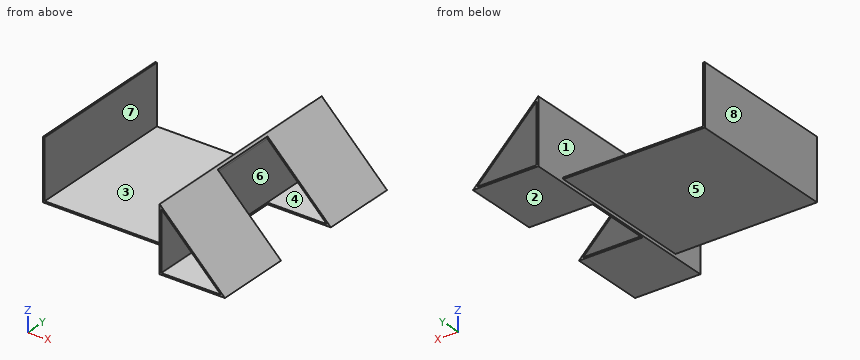
Autodesk Fusion 360 part; units mm, degrees
sketch "Sketch1" plane through (0, 0, 0) normal (0, 1, 0) x (1, 0, 0)
  line L0 (0, 0) -> (-2, 0)
  line L1 (-2, 0) -> (-2, -72)
  line L2 (-2, -72) -> (0, -72)
  line L3 (0, -72) -> (0, 0)
  line L4 (0, 0) -> (166, 0)
  line L5 (166, 0) -> (166, -2)
  line L6 (166, -2) -> (0, -2)
  line L7 (0, -2) -> (0, 0)
  line L8 (166, -72.909) -> (166, 4.011)
  line L9 (166, -72.909) -> (243.52, 4.011)
  line L10 (166, 4.011) -> (243.52, 4.011)
  line L11 (168, -68.107) -> (238.6649, 2.011)
  line L12 (168, 2.011) -> (238.6649, 2.011)
  line L13 (168, -68.107) -> (168, 2.011)
  dimension "d1" = 2
  dimension "d2" = 72
  dimension "d3" = 166
  dimension "d4" = 2
  dimension "d5" = 76.92
  dimension "d6" = 4.011
  dimension "d8" = 77.52
  dimension "d9" = 2
extrude "Extrude1" add sketch "Sketch1" along normal blind 260
sketch "Sketch2" plane through (0, 0, 2) normal (0, 0, 1) x (-1, 0, 0)
  line L0 (0, 0) -> (-166, 0)
  line L1 (-166, 0) -> (-166, -260)
  line L2 (-166, -260) -> (0, -260)
  line L3 (0, -260) -> (0, 0)
  line L4 (2, 0) -> (-166, 0)
  line L5 (-166, 0) -> (-166, -40)
  line L6 (-166, -40) -> (2, -40)
  line L7 (2, -40) -> (2, 0)
  line L8 (0, -130) -> (-166, -130) construction
  line L9 (2, -220) -> (2, -260)
  line L10 (-166, -220) -> (2, -220)
  line L11 (2, -260) -> (-166, -260)
  line L12 (-166, -260) -> (-166, -220)
  point P0 (2, 0)
  dimension "d12" = 168
  dimension "d13" = 40
extrude "Extrude2" cut sketch "Sketch2" against normal blind 45 contours L0 L1 L3 L4 L5 L6 | L3 L4 L6 L7 | L3 L9 L10 L11 | L1 L2 L3 L10 L11 L12
extrude "Extrude3" cut sketch "Sketch2" along normal blind 80 contours L3 L4 L6 L7 | L3 L9 L10 L11
sketch "Sketch3" plane through (0, 0, 2) normal (0, 0, 1) x (-1, 0, 0)
  line L0 (-166, -220) -> (0, -220)
  line L1 (0, -220) -> (0, -40)
  line L2 (0, -40) -> (-166, -40)
  line L3 (-166, -40) -> (-166, -220)
  line L4 (-168.32, -170) -> (-243.52, -170)
  line L5 (-243.52, -170) -> (-243.52, -90)
  line L6 (-243.52, -90) -> (-168.32, -90)
  line L7 (-168.32, -90) -> (-168.32, -170)
  line L8 (-243.52, 0) -> (-243.52, -260)
  dimension "d18" = 75.2
  dimension "d19" = 80
extrude "Extrude4" cut sketch "Sketch3" along normal mid plane 260 contours L4 L5 L6 L7 L8
equation "d2 = ( 7.2 * 10 ) * 1 mm"
equation "d3 = ( 16.6 * 10 ) * 1 mm"
Model file for the job. Use its own axes, mm. Face numbers are marked on the shaded views. A direction names the side the tool comes from. Give positions to 0.01 mm unless a question says otherwise; leave off trailing zeros. Loops run counter-clockwise (first coordinate to the right, second up) from the corner with the lowest first, then second, coordinate; pieces in that order, holes last. Notation, with made-up numbers: (70.25, 88) -> (86.25, 88) arc R20 cw to (86.25, 105) -> close; hole circle Ø8 at (-37, 62). An arc over 180 degrees is marked (long way). Use a Markdown table: item, result. Add a question column.
(1) Tool access for the marked faces 5, 6, 7 and 8: list every direction of +Z, -Z, +X, -X, +Y, -Y with a clear straight run to the whole face (end or side of a thin tool).
(2) Drop flat-ended pins along their axis: pin 1 Ø1 at (y, z) = (100, 9) entering from +X; pin 2 Ø1 at (x, y) = (-1, 114.5) entering from +Z; pin 3 Ø1 at (y, z) = (119, -3) entering from +X; pin 4 Ø22.5 at (x, z) = (213.5, 30) entering from +Y. Give the stop position or say it passes through.
(3) Slice it at A-A on y = 43. List the corners of the cut face in (x, z), and give its area (3 significant figures).
(4) Mould opens along Z. For the marked faces 1, 2, 3 and 4 say: +Z half, -Z half, draft (parallel to the pull), parting line (faces both ways), or undercut.
(5) Slice it at D-D on y = 98.5. List the corners of the cut face in (x, z).
(6) Slice it at C-C on x = 201.5. List the corners of the cut face in (y, z), and give its area (3 significant figures).
(7) Wall check: line 1 along Y through (x, z) = (200, 38); line 2 along X through (y, z) = (93, 29.5); line 3 along Z through (x, y) = (180.5, 68). Give the ranges that are in metal, low to high.
(8) Slice it at B-B on z = 51. List the corners of the cut face in (x, y), and give its area (3 significant figures).
Filled sheet:
| question | item | result |
|---|---|---|
| 1 | face 5 | -Z, -X, +Y, -Y |
| 1 | face 6 | +Y, -Y |
| 1 | face 7 | +Z, +Y, -Y |
| 1 | face 8 | +Z, -Z, -X, +Y, -Y |
| 2 | pin 1 | x = 168 |
| 2 | pin 2 | z = 72 |
| 2 | pin 3 | x = 168.32 |
| 2 | pin 4 | y = 260 |
| 3 | outline | (-2, 0) -> (166, 0) -> (166, -4.01) -> (243.52, -4.01) -> (166, 72.91) -> (166, 2) -> (0, 2) -> (0, 72) -> (-2, 72) -> close; hole (168, -2.01) -> (238.66, -2.01) -> (168, 68.11) -> close |
| 3 | area | 980 mm2 |
| 4 | face 1 | draft |
| 4 | face 2 | -Z half |
| 4 | face 3 | +Z half |
| 4 | face 4 | undercut |
| 5 | outline | (-2, 0) -> (166, 0) -> (166, -4.01) -> (168.32, -4.01) -> (168.32, -2.01) -> (168, -2.01) -> (168, 68.11) -> (168.32, 67.79) -> (168.32, 70.61) -> (166, 72.91) -> (166, 2) -> (0, 2) -> (0, 72) -> (-2, 72) -> close |
| 6 | outline | (0, -4.01) -> (90, -4.01) -> (90, -2.01) -> (0, -2.01) -> close; (0, 34.87) -> (90, 34.87) -> (90, 37.68) -> (0, 37.68) -> close; (170, -4.01) -> (260, -4.01) -> (260, -2.01) -> (170, -2.01) -> close; (170, 34.87) -> (260, 34.87) -> (260, 37.68) -> (170, 37.68) -> close |
| 6 | area | 867 mm2 |
| 7 | line 1 | 0 to 90, 170 to 260 |
| 7 | line 2 | -2 to 0, 166 to 168 |
| 7 | line 3 | -4.01 to -2.01, 55.7 to 58.52 |
| 8 | outline | (-2, 40) -> (0, 40) -> (0, 220) -> (-2, 220) -> close; (166, 0) -> (168, 0) -> (168, 260) -> (166, 260) -> close; (185.24, 0) -> (188.08, 0) -> (188.08, 90) -> (185.24, 90) -> close; (185.24, 170) -> (188.08, 170) -> (188.08, 260) -> (185.24, 260) -> close |
| 8 | area | 1,390 mm2 |
